```python
from build123d import *

# Parameters (mm, degrees)
PAD_DEPTH    = 8
SKETCH001_W  = 27.8
SKETCH001_H  = 1.7
POCKET_DEPTH = 4
CHAMFER_SIZE = 0.5


with BuildPart() as part:
    # Sketch → Pad (new body)
    with BuildSketch(Plane.XY):
        Polygon((-13.9, 0), (-13.9, 13.2), (-9.9, 13.2), (-9.9, 11.2), (-11.9, 11.2), (-11.9, 9.5), (11.9, 9.5), (11.9, 11.2), (9.9, 11.2), (9.9, 13.2), (13.9, 13.2), (13.9, 0), align=None)
    extrude(amount=PAD_DEPTH)

    # Sketch001 → Pocket (cut)
    with BuildSketch(Plane.XY.offset(8)):
        with Locations((0, 2.35)):
            Rectangle(SKETCH001_W, SKETCH001_H)
    extrude(amount=-POCKET_DEPTH, mode=Mode.SUBTRACT)

    # Chamfer
    chamfer_edges = [part.edges().sort_by_distance(p)[0] for p in [
        (0, 1.5, 8),
        (0, 3.2, 8),
        (0, 9.5, 8),
        (-11.9, 10.35, 8),
        (-10.9, 11.2, 8),
        (11.9, 10.35, 8),
        (10.9, 11.2, 8),
        (-13.9, 13.2, 4),
        (13.9, 13.2, 4),
    ]]
    chamfer(chamfer_edges, length=CHAMFER_SIZE)


solid = part.part
```
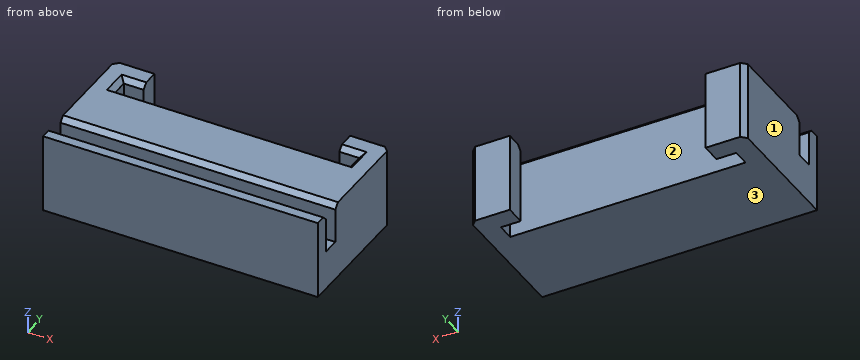
CAD build for the part. Positions are in the model's coordinates, mm. Face numbers are marked on the shaded views. Round coordinates to 2 decimals unless told otherwise and drop trailing zeros. Order: outer loops, then holes, each group sorted by start corner. A loop starts at its lowest first (then second) coordinate and runs counter-clockwise, first axis right, second up.
Q1. Slice it at D-D (z = 2). Write the cut outline in (x, y).
Q2. Two-plate mould, pull along X, no slides. Class the marked faces 1, 2 and 3: pulls with the +X half, pulls with the -X half, needs draft (parallel to the pull), parting line crosses it, or undercut.
Q3. Wall check: L1, parallel to Y at x = -10.5, z = 5.5; L2, parallel to Y at x = 1.5, z = 4.5; L3, parallel to X at y = 10.25, z = 1.75. Give the ranges that are in metal, low to high.
Q4. Slice it at C-C (y = 12.25). Write the cut outline in (x, z).
Q5. Drop flat-ended pins along their axis: pin 1 (1.5 mm diameter, centred on x = 1.5, y = 11, fed in from +Z); pin 2 (3 mm diameter, centred on x = -6, z = 5.5, fed in from +Y); pin 3 (0.8 mm diameter, centred on x = -6, y = 2.5, fed in from +Z). Give the stop position or say it passes through.
Q6. Slice it at B-B (x = 11.25). Write the cut outline in (y, z).
Q7. Slice it at A-A (z = 6.75). Write the cut outline in (x, y).
Results below:
1. outline: (-13.9, 0) - (13.9, 0) - (13.9, 12.7) - (13.4, 13.2) - (9.9, 13.2) - (9.9, 11.2) - (11.9, 11.2) - (11.9, 9.5) - (-11.9, 9.5) - (-11.9, 11.2) - (-9.9, 11.2) - (-9.9, 13.2) - (-13.4, 13.2) - (-13.9, 12.7) - close
2. face 1: pulls with the -X half
2. face 2: undercut
2. face 3: needs draft
3. L1: y = 0 to 1.5, 3.2 to 9.5, 11.2 to 13.2
3. L2: y = 0 to 1.5, 3.2 to 9.5
3. L3: x = -13.9 to -11.9, 11.9 to 13.9
4. outline: (-13.9, 0) - (-9.9, 0) - (-9.9, 8) - (-13.9, 8) - close; (9.9, 0) - (13.9, 0) - (13.9, 8) - (9.9, 8) - close
5. pin 1: passes through
5. pin 2: stops at y = 9.5
5. pin 3: stops at z = 4
6. outline: (0, 0) - (9.5, 0) - (9.5, 7.5) - (9, 8) - (3.7, 8) - (3.2, 7.5) - (3.2, 4) - (1.5, 4) - (1.5, 7.5) - (1, 8) - (0, 8) - close; (11.2, 0) - (13.2, 0) - (13.2, 8) - (11.7, 8) - (11.2, 7.5) - close
7. outline: (-13.9, 0) - (13.9, 0) - (13.9, 1.5) - (-13.9, 1.5) - close; (-13.9, 3.2) - (13.9, 3.2) - (13.9, 12.7) - (13.4, 13.2) - (9.9, 13.2) - (9.9, 11.2) - (11.9, 11.2) - (11.9, 9.5) - (-11.9, 9.5) - (-11.9, 11.2) - (-9.9, 11.2) - (-9.9, 13.2) - (-13.4, 13.2) - (-13.9, 12.7) - close
